Verification items for this drawing (mm, ordinates from the low corner). A direction names the side the tool comes from. Coordinates: 2 decimals unless noted, no trailing zeros. Order: outer loops, then holes, each group sorted by start corner. A loop starts at its lowest first (then second) coordinate and runs counter-clockwise, first axis right, second up. Notation, with made-up numbers: M 36.25,-31 L 72.25,-31 A11 cw 72.25,-21 Z; hole C 8.5,50.5 d9. An arc over 180 degrees is marked long. Answer as a JSON object with one key per item and string values. Group by question number.
(1) Material ranges on line 1 (Y direction, x = 30, z = 64.5); line 2 (Z direction, x = 36, y = 40); line 3 (Z direction, x = 45, y = 20), recorded low to high.
(2) Cross-section at B-B (y = 17). Enter the section's corners in (x, z) (1 decimal).
(3) Cross-section at A-A (y = 40). Enter the section's corners in (x, z).
(4) Gauge pin test, flat ends, axial feed: pin 1 Ø10 at (x, y) = (30, 40.5) entering from +Z; pin 2 Ø4 at (x, y) = (15.5, 15) entering from -Z; pin 3 Ø10 at (x, y) = (14.5, 31) entering from +Z (1 decimal). Record the tip position at first contact, or that the pin passes through.
(5) Cross-section at C-C (x = 30). Enter the section's corners in (y, z), plus the area to 3 significant figures.
(6) Access from +Z, -Z, +X, -X, +Y, -Y to the whole of each face (thin tool, end or side, straight path). Record for the marked faces 1, 2 and 3.
(7) Cross-section at D-D (z = 62.5). Enter the section's corners in (x, y), plus the area to 3 significant figures.
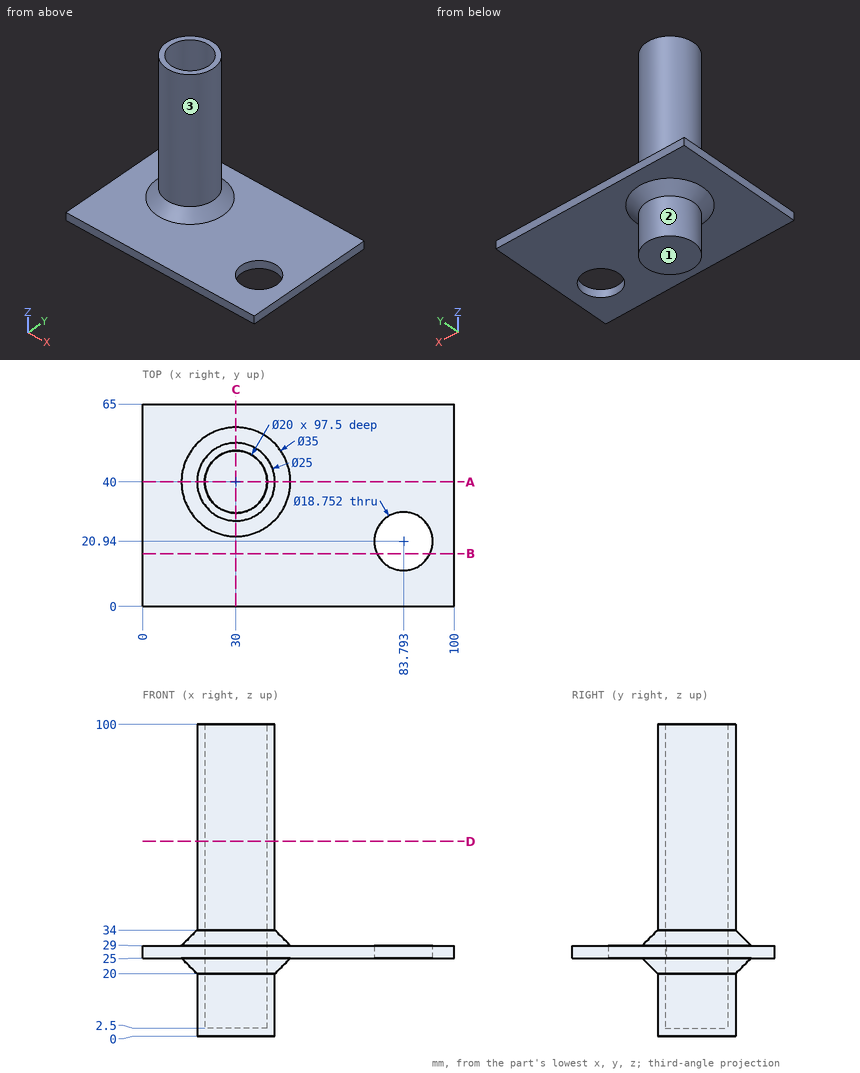
Taken from the geometry:
{
 "1": {"line 1": "y = 27.5 to 30, 50 to 52.5", "line 2": "z = 0 to 2.5", "line 3": "z = 25 to 29"},
 "2": {"outline": "M 0,25 L 75.3,25 L 75.3,29 L 0,29 Z; M 92.3,25 L 100,25 L 100,29 L 92.3,29 Z"},
 "3": {"outline": "M 0,25 L 12.5,25 L 17.5,20 L 17.5,0 L 42.5,0 L 42.5,20 L 47.5,25 L 100,25 L 100,29 L 47.5,29 L 42.5,34 L 42.5,100 L 40,100 L 40,2.5 L 20,2.5 L 20,100 L 17.5,100 L 17.5,34 L 12.5,29 L 0,29 Z"},
 "4": {"pin 1": "stops at z = 2.5", "pin 2": "stops at z = 25", "pin 3": "stops at z = 33.6"},
 "5": {"outline": "M 0,25 L 22.5,25 L 27.5,20 L 27.5,0 L 52.5,0 L 52.5,20 L 57.5,25 L 65,25 L 65,29 L 57.5,29 L 52.5,34 L 52.5,100 L 50,100 L 50,2.5 L 30,2.5 L 30,100 L 27.5,100 L 27.5,34 L 22.5,29 L 0,29 Z", "area": "760 mm²"},
 "6": {"face 1": "-Z, +X, -X, +Y, -Y", "face 2": "-Z", "face 3": "+Z"},
 "7": {"outline": "C 30,40 d25; hole C 30,40 d20", "area": "177 mm²"}
}
